Could you check a few things on this model? Use its own coordinates, in mm. Round coordinates to 2 decimals unless told otherwise and drop trailing zeros. Write each loop counter-clockwise with the first axis right and the second up, starting at its lowest first coordinate (ties: lowest second). Pieces come first, ordered by that corner, then holes. Notation, with made-up numbers: (-13, -25) -> (-2, -25) arc R22 ccw to (-2, 14) -> close; hole circle Ø7 at (-16, 36). An arc over 180 degrees is marked (long way). Return JSON: item names as keys, results as strings.
from build123d import *

# Parameters (mm, degrees)
F1_DEPTH = 500
F2_R     = 4
F3_R     = 3.4
F4_DEPTH = 1000


with BuildPart() as f1:
    # F0 (on Front) → F1 (new body, symmetric)
    with BuildSketch(Plane.XZ):
        Polygon((20, 4), (20, 20), (4, 20), (4, 7.75), (-4, 7.75), (-4, 20), (-20, 20), (-20, 4), (-7.75, 4), (-7.75, -4), (-20, -4), (-20, -20), (-4, -20), (-4, -7.75), (4, -7.75), (4, -20), (20, -20), (20, -4), (7.75, -4), (7.75, 4), align=None)
    extrude(amount=F1_DEPTH, both=True)

    # F2
    f2_edges = [f1.edges().sort_by_distance(p)[0] for p in [
        (-20, 0, 20),
        (20, 0, 20),
        (20, 0, -20),
        (-20, 0, -20),
    ]]
    fillet(f2_edges, radius=F2_R)

    # F3 (on face) → F4 (cut)
    with BuildSketch(Plane.XZ.offset(500)):
        Circle(F3_R)
    extrude(amount=-F4_DEPTH, mode=Mode.SUBTRACT)


solid = f1.part
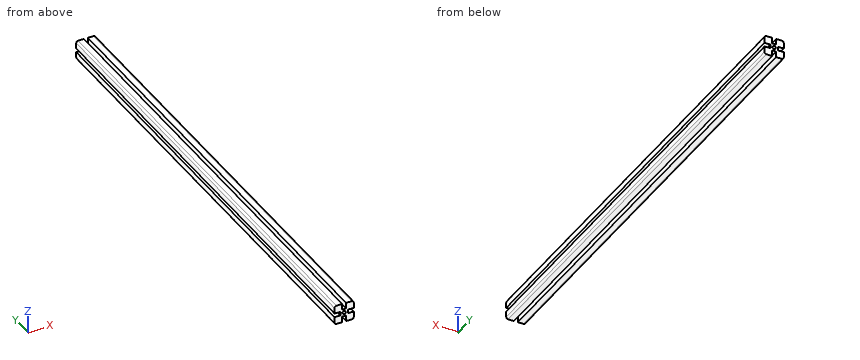
1) I want a section at A-A, the plane y = 255. Please give me the cut outline in (x, z).
Return value:
{"outline": "(-20, -16) arc R4 ccw to (-16, -20) -> (-4, -20) -> (-4, -7.75) -> (4, -7.75) -> (4, -20) -> (16, -20) arc R4 ccw to (20, -16) -> (20, -4) -> (7.75, -4) -> (7.75, 4) -> (20, 4) -> (20, 16) arc R4 ccw to (16, 20) -> (4, 20) -> (4, 7.75) -> (-4, 7.75) -> (-4, 20) -> (-16, 20) arc R4 ccw to (-20, 16) -> (-20, 4) -> (-7.75, 4) -> (-7.75, -4) -> (-20, -4) -> close; hole circle Ø6.8 at (0, 0)"}
2) Will these pins go through, and if not, where does the flat tip stop? pin 1 Ø4 at (x, y) = (1.5, -366.5) entering from -Z; pin 2 Ø4 at (y, z) = (360, 1) entering from -X; pin 3 Ø4 at (x, z) = (0, 0) entering from -Y; pin 4 Ø6.5 at (y, z) = (50, 0) entering from +X.
Return value:
{"pin 1": "z = -7.75", "pin 2": "x = -7.75", "pin 3": "through", "pin 4": "x = 7.75"}
3) If I drill on probe 1 along Z at (x, y) = (8, -237.5); probe 2 along Z at (x, y) = (0, -228), over which ranges is the centre line in solid material (lowest first)? Write a range as [from, to].
Return value:
{"probe 1": "[-20, -4], [4, 20]", "probe 2": "[-7.75, -3.4], [3.4, 7.75]"}
